from build123d import *
from OCP.BRepFilletAPI import BRepFilletAPI_MakeChamfer

# Parameters (mm, degrees)
BOSS_EXTRUDE1_DEPTH                                 = 4.5
BOSS_EXTRUDE2_REACH                                 = 32.037
BOSS_EXTRUDE2_END_RADIUS                            = 21
BOSS_EXTRUDE2_DIRECTION_2_REACH                     = 32.037
BOSS_EXTRUDE2_DIRECTION_2_END_RADIUS                = 21
CUT_EXTRUDE1_REACH                                  = 32.037
CUT_EXTRUDE1_DIRECTION_2_REACH                      = 32.037
CBORE_FOR_M3_HEX_SOCKET_HEAD_CAP_SCREW1_D           = 3.8
CBORE_FOR_M3_HEX_SOCKET_HEAD_CAP_SCREW1_DEPTH       = 7
CBORE_FOR_M3_HEX_SOCKET_HEAD_CAP_SCREW1_CBORE_D     = 6.5
CBORE_FOR_M3_HEX_SOCKET_HEAD_CAP_SCREW1_CBORE_DEPTH = 2.9
CBORE_FOR_M3_HEX_SOCKET_HEAD_CAP_SCREW1_TIP         = 1.141635176
CHAMFER1_SIZE                                       = 3
CHAMFER1_SIZE2                                      = 4.28444402
CHAMFER2_SIZE                                       = 3


with BuildPart() as part:
    # Sketch1 → Boss-Extrude1 (new body)
    with BuildSketch(Plane(origin=(0, 0, 0), x_dir=(0, 0, -1), z_dir=(1, 0, 0))):
        with BuildLine():
            Line((-6, -10.5), (-6, 0))
            ThreePointArc((-6, 0), (0, 6), (6, 0))
            Line((6, 0), (6, -10.5))
            Line((6, -10.5), (18.186533479, -10.5))
            ThreePointArc((18.186533479, -10.5), (0, 21), (-18.186533479, -10.5))
            Line((-18.186533479, -10.5), (-6, -10.5))
        make_face()
    extrude(amount=BOSS_EXTRUDE1_DEPTH)

    # Boss-Extrude2: up to this cylinder (the profile starts inside it)
    boss_extrude2_end = Plane(origin=(1.5, 0, 0), z_dir=(-1, 0, 0)) * Cylinder(BOSS_EXTRUDE2_END_RADIUS, 107.074, mode=Mode.PRIVATE)
    # Sketch2 → Boss-Extrude2 (add, up to the surface)
    with BuildSketch(Plane.XY, mode=Mode.PRIVATE) as boss_extrude2_sk1:
        Polygon((4.5, -10.5), (0, -15), (0, -10.5), align=None)
    boss_extrude2_tool1 = extrude(boss_extrude2_sk1.sketch, amount=-BOSS_EXTRUDE2_REACH, mode=Mode.PRIVATE) & boss_extrude2_end
    add(boss_extrude2_tool1.solids().sort_by_distance((1.5, -12, 0))[0])

    # Boss-Extrude2 direction 2: up to this cylinder (the profile starts inside it)
    boss_extrude2_direction_2_end = Plane(origin=(1.5, 0, 0), z_dir=(-1, 0, 0)) * Cylinder(BOSS_EXTRUDE2_DIRECTION_2_END_RADIUS, 107.074, mode=Mode.PRIVATE)
    # Sketch2 → Boss-Extrude2 direction 2 (add, up to the surface)
    with BuildSketch(Plane.XY, mode=Mode.PRIVATE) as boss_extrude2_direction_2_sk1:
        Polygon((4.5, -10.5), (0, -15), (0, -10.5), align=None)
    boss_extrude2_direction_2_tool1 = extrude(boss_extrude2_direction_2_sk1.sketch, amount=BOSS_EXTRUDE2_DIRECTION_2_REACH, mode=Mode.PRIVATE) & boss_extrude2_direction_2_end
    add(boss_extrude2_direction_2_tool1.solids().sort_by_distance((1.5, -12, 0))[0])

    # Cut-Extrude1: up to this face of the body (flat: up to its plane)
    cut_extrude1_end = Plane(part.part.faces().sort_by_distance((2.25, -5.25, -6))[0])
    # Sketch2<2> → Cut-Extrude1 (cut, up to the picked face)
    with BuildSketch(Plane.XY, mode=Mode.PRIVATE) as cut_extrude1_sk1:
        Polygon((4.5, -10.5), (0, -15), (0, -10.5), align=None)
    cut_extrude1_tool1 = split(extrude(cut_extrude1_sk1.sketch, amount=-CUT_EXTRUDE1_REACH, mode=Mode.PRIVATE), bisect_by=cut_extrude1_end, keep=Keep.BOTH, mode=Mode.PRIVATE)
    add(cut_extrude1_tool1.solids().sort_by(Axis((1.5, -12, 0), (0, 0, -1)))[0], mode=Mode.SUBTRACT)

    # Cut-Extrude1 direction 2: up to this face of the body (flat: up to its plane)
    cut_extrude1_direction_2_end = Plane(part.part.faces().sort_by_distance((2.25, -5.25, 6))[0])
    # Sketch2<2> → Cut-Extrude1 direction 2 (cut, up to the picked face)
    with BuildSketch(Plane.XY, mode=Mode.PRIVATE) as cut_extrude1_direction_2_sk1:
        Polygon((4.5, -10.5), (0, -15), (0, -10.5), align=None)
    cut_extrude1_direction_2_tool1 = split(extrude(cut_extrude1_direction_2_sk1.sketch, amount=CUT_EXTRUDE1_DIRECTION_2_REACH, mode=Mode.PRIVATE), bisect_by=cut_extrude1_direction_2_end, keep=Keep.BOTH, mode=Mode.PRIVATE)
    add(cut_extrude1_direction_2_tool1.solids().sort_by(Axis((1.5, -12, 0), (0, 0, 1)))[0], mode=Mode.SUBTRACT)

    # CBORE for M3 Hex Socket Head Cap Screw1
    with Locations(Plane(origin=(4.5, 0, 0), x_dir=(0, 0, -1), z_dir=(1, 0, 0))):
        with Locations((-17.5, 0), (17.5, 0)):
            CounterBoreHole(CBORE_FOR_M3_HEX_SOCKET_HEAD_CAP_SCREW1_D / 2, CBORE_FOR_M3_HEX_SOCKET_HEAD_CAP_SCREW1_CBORE_D / 2, CBORE_FOR_M3_HEX_SOCKET_HEAD_CAP_SCREW1_CBORE_DEPTH, depth=CBORE_FOR_M3_HEX_SOCKET_HEAD_CAP_SCREW1_DEPTH)
            with Locations((0, 0, -(CBORE_FOR_M3_HEX_SOCKET_HEAD_CAP_SCREW1_DEPTH + CBORE_FOR_M3_HEX_SOCKET_HEAD_CAP_SCREW1_TIP / 2))):  # 118° drill point
                Cone(0, CBORE_FOR_M3_HEX_SOCKET_HEAD_CAP_SCREW1_D / 2, CBORE_FOR_M3_HEX_SOCKET_HEAD_CAP_SCREW1_TIP, mode=Mode.SUBTRACT)

    # Chamfer1: one chamfer whose edges measure the first distance from different faces: ONE call of the kernel's chamfer builder (chamfer() names one face for all edges)
    chamfer1_edges_1 = [part.edges().sort_by_distance(p)[0] for p in [
        (4.5, -5.25, 6),
    ]]
    chamfer1_side_1 = [part.faces().sort_by_distance(p)[0] for p in [
        (2.117647059, -6.441176471, 6),
    ]]
    chamfer1_edges_2 = [part.edges().sort_by_distance(p)[0] for p in [
        (4.5, 6, 0),
    ]]
    chamfer1_side_2 = [part.faces().sort_by_distance(p)[0] for p in [
        (2.25, 6, 0),
    ]]
    chamfer1_edges_3 = [part.edges().sort_by_distance(p)[0] for p in [
        (4.5, -5.25, -6),
    ]]
    chamfer1_side_3 = [part.faces().sort_by_distance(p)[0] for p in [
        (2.117647059, -6.441176471, -6),
    ]]
    chamfer1 = BRepFilletAPI_MakeChamfer(part.part.solid().wrapped)
    for e in chamfer1_edges_1:
        chamfer1.Add(CHAMFER1_SIZE, CHAMFER1_SIZE2, e.wrapped, chamfer1_side_1[0].wrapped)  # the first distance lies on this face
    for e in chamfer1_edges_2:
        chamfer1.Add(CHAMFER1_SIZE, CHAMFER1_SIZE2, e.wrapped, chamfer1_side_2[0].wrapped)  # the first distance lies on this face
    for e in chamfer1_edges_3:
        chamfer1.Add(CHAMFER1_SIZE, CHAMFER1_SIZE2, e.wrapped, chamfer1_side_3[0].wrapped)  # the first distance lies on this face
    add(Compound.cast(chamfer1.Shape()), mode=Mode.REPLACE)

    # Chamfer2
    # the kernel refuses this chamfer: 3 mm, written as the material it takes off along each edge
    with BuildSketch(Plane(origin=(4.5, 0, 0), x_dir=(0, -0.7783499423883817, -0.6278306835317966), z_dir=(0, -0.6278306835317966, 0.7783499423883817))) as chamfer2_piece_1:
        Polygon((21 - CHAMFER2_SIZE, 0), (21, -CHAMFER2_SIZE), (21, 0), align=None)
    revolve(axis=Axis((4.5, 0, 0), (1, 0, 0)), revolution_arc=282.219489944, mode=Mode.SUBTRACT)


solid = part.part
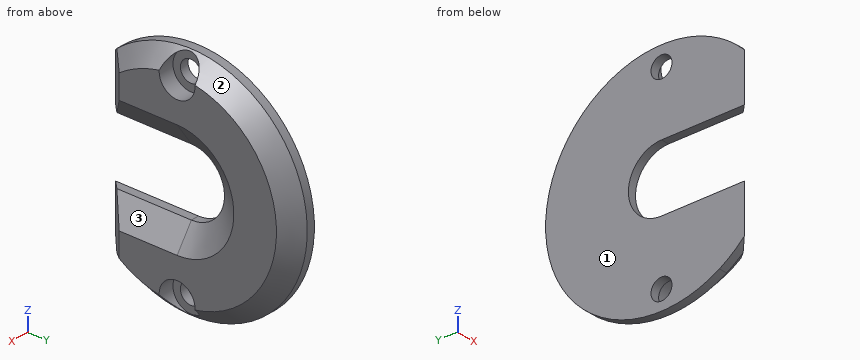
Input: part model. Units: mm. Frame: model coordinates. Face numbers are marked on the shaded views. Give positions to 0.01 mm unless a question says otherwise; leave off trailing zeros. Loops run counter-clockwise (first coordinate to the right, second up) from the corner with the lowest first, then second, coordinate; pieces in that order, holes last. Notation, with made-up numbers: (79.5, 5.25) -> (117.5, 5.25) arc R30 cw to (117.5, 32.25) -> close; hole circle Ø8 at (60.25, 57.5). An arc over 180 degrees is marked (long way). Answer as a JSON object with one key per item and string values. Group by question number.
Item 1: Pull-direction query (Z, two-part tool) for the marked faces 1, 2 and 3; classes: released by +Z, released by -Z, zero draft, split by the parting line, or undercut.
Item 2: Cut plane A-A, the plane x = 2.9. Return the cut outline in (y, z).
Item 3: Cut plane C-C, the plane z = 0. Return the cut outline in (x, y), and give its area (3 significant figures).
Item 4: Line query: probe 1 along Z at (x, y) = (3.1, 0); probe 2 along Z at (x, y) = (3, 0); probe 3 along Y at (x, z) = (0.3, -10.5). Output: solid intervals per line, ascending.
Item 5: Pin query (flat end, axial travel): P1, Ø1, axis at x = 0.5, y = 2.5, coming from the +Z side; P2, Ø1.7, axis at x = 1, y = -8.5, coming from the +Z side; P3, Ø0.8, axis at x = 0.5, y = -7.5, coming from the -Z side. Return the tip coordinate at first contact, or that it passes through.
Item 6: Cut plane B-B, the plane x = 0.55. Return the cut outline in (y, z), and give its area (3 significant figures).
Checks:
{
 "1": {"face 1": "zero draft", "face 2": "split by the parting line", "face 3": "undercut"},
 "2": {"outline": "(-12.1, -15.42) arc R19.6 ccw to (-2.62, -19.42) arc R3.25 cw (long way) to (2.62, -19.42) arc R19.6 ccw to (2.62, 19.42) arc R3.25 cw (long way) to (-2.62, 19.42) arc R19.6 ccw to (-12.1, 15.42) -> (-12.1, 8) -> (0, 8) arc R8 cw to (0, -8) -> (-12.1, -8) -> close"},
 "3": {"outline": "(0, 6) -> (1.5, 6) -> (4.5, 10.28) -> (4.5, 18) -> (1.5, 21) -> (0, 21) -> close", "area": "56.6 mm²"},
 "4": {"probe 1": "z = -14.25 to -8.29, 8.29 to 14.25", "probe 2": "z = -14.25 to -8.14, 8.14 to 14.25", "probe 3": "y = -14.7 to 18.19"},
 "5": {"P1": "stops at z = 20.9", "P2": "stops at z = 19.56", "P3": "stops at z = -19.76"},
 "6": {"outline": "(-14.45, -15.24) arc R21 ccw (long way) to (-14.45, 15.24) -> (-14.45, 6) -> (0, 6) arc R6 cw to (0, -6) -> (-14.45, -6) -> close; hole circle Ø3.8 at (0, -17.5); hole circle Ø3.8 at (0, 17.5)", "area": "995 mm²"}
}
